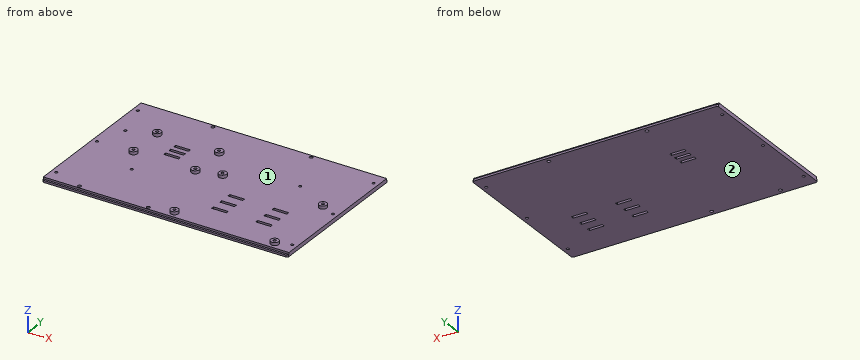
```python
from build123d import *

# Parameters (mm, degrees)
SKETCH_W        = 250
SKETCH_H        = 160
PAD_DEPTH       = 4
SKETCH001_R     = 4
PAD001_DEPTH    = 3
SKETCH002_R     = 1.4
POCKET_DEPTH    = 5
SKETCH019_R     = 1.4
POCKET009_DEPTH = 2
SKETCH022_R     = 1.4
SKETCH022_R_2   = 1.75
SKETCH022_W     = 15
SKETCH022_H     = 3
POCKET010_DEPTH = 5
SKETCH043_W     = 2
SKETCH043_H     = 2
POCKET025_DEPTH = 250.001
CHAMFER032_SIZE = 1.5


with BuildPart() as part:
    # Sketch → Pad (new body)
    with BuildSketch(Plane.XY):
        Rectangle(SKETCH_W, SKETCH_H)
    extrude(amount=PAD_DEPTH)

    # Sketch001 (on Face6 of Pad) → Pad001 (join)
    with BuildSketch(Plane.XY.offset(4)):
        with Locations((4, 6)):
            Circle(SKETCH001_R)
        with Locations((106, 6)):
            Circle(SKETCH001_R)
        with Locations((106, -71)):
            Circle(SKETCH001_R)
        with Locations((4, -71)):
            Circle(SKETCH001_R)
        with Locations((-83.0000000001, 38)):
            Circle(SKETCH001_R)
        with Locations((-20, 38)):
            Circle(SKETCH001_R)
        with Locations((-20, 0)):
            Circle(SKETCH001_R)
        with Locations((-83.0000000001, 0)):
            Circle(SKETCH001_R)
    extrude(amount=PAD001_DEPTH)

    # Sketch002 → Pocket (cut)
    with BuildSketch(Plane.XY.offset(7)):
        with Locations((-83, 38)):
            Circle(SKETCH002_R)
        with Locations((-20, 38)):
            Circle(SKETCH002_R)
        with Locations((-83, 0)):
            Circle(SKETCH002_R)
        with Locations((-20, 0)):
            Circle(SKETCH002_R)
        with Locations((4, 6)):
            Circle(SKETCH002_R)
        with Locations((106, 6)):
            Circle(SKETCH002_R)
        with Locations((106, -71)):
            Circle(SKETCH002_R)
        with Locations((4, -71)):
            Circle(SKETCH002_R)
    extrude(amount=-POCKET_DEPTH, mode=Mode.SUBTRACT)

    # Sketch019 (on Face5 of Pocket) → Pocket009 (cut)
    with BuildSketch(Plane.XY.offset(4)):
        with Locations((-110, 29.3395385444)):
            Circle(SKETCH019_R)
        with Locations((69.686069743, 26.5638621346)):
            Circle(SKETCH019_R)
        with Locations((-68.3727818418, -25.7609993889)):
            Circle(SKETCH019_R)
    extrude(amount=-POCKET009_DEPTH, mode=Mode.SUBTRACT)

    # Sketch022 (on Face5 of Pocket009) → Pocket010 (cut)
    with BuildSketch(Plane.XY.offset(4)):
        with Locations((-120, 65)):
            Circle(SKETCH022_R)
        with Locations((-120, -65)):
            Circle(SKETCH022_R)
        with Locations((120, 65)):
            Circle(SKETCH022_R)
        with Locations((120, -65)):
            Circle(SKETCH022_R)
        with Locations((-50, 75)):
            Circle(SKETCH022_R_2)
        with Locations((50, 75)):
            Circle(SKETCH022_R_2)
        with Locations((-90, -75)):
            Circle(SKETCH022_R_2)
        with Locations((-20, -75)):
            Circle(SKETCH022_R_2)
        with Locations((-120, 0)):
            Circle(SKETCH022_R)
        with Locations((120, 0)):
            Circle(SKETCH022_R)
        with Locations((34.2977322278, -19.8916100594)):
            Rectangle(SKETCH022_W, SKETCH022_H)
        with Locations((34.2977322278, -32.8916100594)):
            Rectangle(SKETCH022_W, SKETCH022_H)
        with Locations((34.2977322278, -45.8916100594)):
            Rectangle(SKETCH022_W, SKETCH022_H)
        with Locations((79.2977322278, -19.8916100594)):
            Rectangle(SKETCH022_W, SKETCH022_H)
        with Locations((79.2977322278, -32.8916100594)):
            Rectangle(SKETCH022_W, SKETCH022_H)
        with Locations((79.2977322278, -45.8916100594)):
            Rectangle(SKETCH022_W, SKETCH022_H)
        with Locations((-51.8112448514, 28.8282704754)):
            Rectangle(SKETCH022_W, SKETCH022_H)
        with Locations((-51.8112448514, 20.8282704754)):
            Rectangle(SKETCH022_W, SKETCH022_H)
        with Locations((-51.8112448514, 12.8282704754)):
            Rectangle(SKETCH022_W, SKETCH022_H)
    extrude(amount=-POCKET010_DEPTH, mode=Mode.SUBTRACT)

    # Sketch043 (on Face2 of Pocket010) → Pocket025 (cut, through all)
    with BuildSketch(Plane(origin=(-125, 0, 0), x_dir=(0, -1, 0), z_dir=(-1, 0, 0))):
        with Locations((79, 3)):
            Rectangle(SKETCH043_W, SKETCH043_H)
        with Locations((-79, 3)):
            Rectangle(SKETCH043_W, SKETCH043_H)
    extrude(amount=-POCKET025_DEPTH, mode=Mode.SUBTRACT)

    # Chamfer032
    chamfer032_edges = [part.edges().sort_by_distance(p)[0] for p in [
        (-125, 80, 1),
        (125, 80, 1),
        (125, -80, 1),
        (-125, -80, 1),
    ]]
    chamfer(chamfer032_edges, length=CHAMFER032_SIZE)


with BuildPart() as part_1:
    # Body placement: moved
    add(part.part.moved(Location((0, 0, -36.5))))


solid = part_1.part
```
Work out the finished part from the listing and answer in its coordinate system (mm). Face numbers are marked on the shaded views. A direction names the side the tool comes from. Give positions to 0.01 mm unless a question says otherwise; leave off trailing zeros. Loops run counter-clockwise (first coordinate to the right, second up) from the corner with the lowest first, then second, coordinate; pieces in that order, holes last. Notation, with made-up numbers: (35.5, -39) -> (72.5, -39) arc R17 ccw to (72.5, -6) -> close; hole circle Ø7 at (9, 32.5). An arc over 180 degrees is marked (long way). One line per question, with ' | ' between items. Start each with the question number.
1) Section B-B, the plane y = -15.5 is taken. Determine the outline of the cut face in (x, z), then the cut area to 3 significant figures.
2) Section A-A, the plane x = 79 is taken. Determine the outline of the cut face in (y, z).
3) Straight lines are drawn through the part: L1, parallel to Y at x = 120, z = -34; L2, parallel to Y at x = -120, z = -35.2; L3, parallel to X at y = -19, z = -34. For each, find the intervals that lie inside material, in ascending order.
4) For the marked faces 1 and 2, determine the directions among +Z, -Z, +X, -X, +Y, -Y from which every point of the face is accessible in a straight line to the end or side of a thin tool.
5) Each of these flat-tipped pins is pushed along its axis until it touches: pin 1 (3.5 mm diameter, centred on x = -68.37, y = -25.76, fed in from +Z); pin 2 (2 mm diameter, centred on x = 70, y = 26.5, fed in from +Z). Where does it stop, or does it pass through?
Resolved:
1) outline: (-125, -36.5) -> (125, -36.5) -> (125, -32.5) -> (-125, -32.5) -> close | area: 1,000 mm2
2) outline: (-80, -36.5) -> (-47.39, -36.5) -> (-47.39, -32.5) -> (-78, -32.5) -> (-78, -34.5) -> (-80, -34.5) -> close; (-44.39, -36.5) -> (-34.39, -36.5) -> (-34.39, -32.5) -> (-44.39, -32.5) -> close; (-31.39, -36.5) -> (-21.39, -36.5) -> (-21.39, -32.5) -> (-31.39, -32.5) -> close; (-18.39, -36.5) -> (80, -36.5) -> (80, -34.5) -> (78, -34.5) -> (78, -32.5) -> (-18.39, -32.5) -> close
3) L1: -78 to -66.4, -63.6 to -1.4, 1.4 to 63.6, 66.4 to 78 | L2: -80 to -66.4, -63.6 to -1.4, 1.4 to 63.6, 66.4 to 80 | L3: -125 to 26.8, 41.8 to 71.8, 86.8 to 125
4) face 1: +Z | face 2: -Z, +X, -X, +Y, -Y
5) pin 1: z = -32.5 | pin 2: z = -34.5
